Work out the finished part from the listing and answer in its coordinate system (mm). Face numbers are marked on the shaded views. Round coordinates to 2 decimals unless told otherwise and drop trailing zeros. Loops run counter-clockwise (first coordinate to the right, second up) from the corner with the lowest first, then second, coordinate; pieces in that order, holes last.
Autodesk Inventor part; units mm, degrees
ref_plane "YZ Plane" through (0, 0, 0) normal (1, 0, 0) x (0, 1, 0)
ref_plane "XZ Plane" through (0, 0, 0) normal (0, 1, 0) x (-1, 0, 0)
ref_plane "XY Plane" through (0, 0, 0) normal (0, 0, 1) x (1, 0, 0)
sketch "Sketch1" plane through (0, 0, 0) normal (0, 1, 0) x (-1, 0, 0)
  line L0 (-12.5, -5) -> (12.5, -5)
  line L1 (12.5, 0) -> (12.5, 0)
  line L2 (12.5, 5) -> (-12.5, 5)
  line L3 (-12.5, 0) -> (-12.5, 0)
  line L4 (-12.5, -5) -> (12.5, 5) construction
  line L5 (12.5, -5) -> (-12.5, 5) construction
  circle A0 centre (10, 0) radius 1
  circle A1 centre (0, 0) radius 2.5
  line L6 (-12.5, 5) -> (-12.5, -5)
  line L7 (12.5, 5) -> (12.5, -5)
  circle A2 centre (-10, 0) radius 1
  point P0 (0, 0)
  dimension "d0" = 10
  dimension "d1" = 25
  dimension "d3" = 2
  dimension "d4" = 5
  dimension "d6" = 2.5
  dimension "d7" = 5
  dimension "d8" = 5
  dimension "d12" = 0
  dimension "d13" = 2
  dimension "d14" = 2.5
  dimension "d15" = 5
extrude "Extrusion1" add sketch "Sketch1" along normal blind 5
properties part number "link"
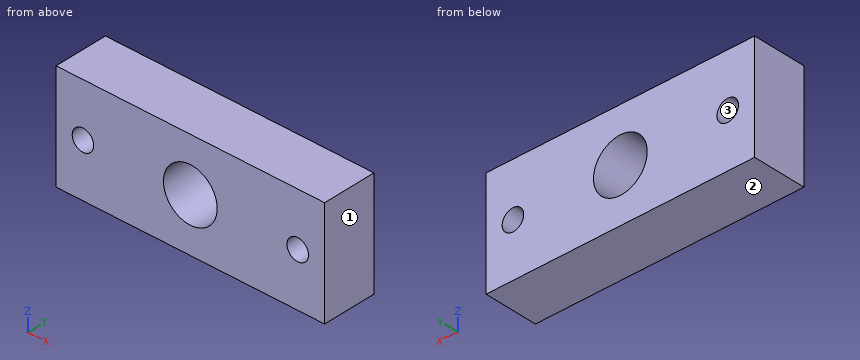
1. Consider probe 1 along Z at (x, y) = (10, 3.55); probe 2 along Z at (x, y) = (0, 1.4); probe 3 along X at (y, z) = (0.4, -2). Determine where each line is inside the solid, lowest interval first.
Answer key:
probe 1: z = -5 to -1, 1 to 5
probe 2: z = -5 to -2.5, 2.5 to 5
probe 3: x = -12.5 to -1.5, 1.5 to 12.5
2. Determine the mould class of the marked faces 1, 2 and 3 for opening direction X: +X half, -X half, draft (parallel to the pull), parting line (faces both ways), or undercut.
Answer key:
face 1: +X half
face 2: draft
face 3: undercut
3. Find section D-D (z = 1.25). Write down the section's boundary in (x, y).
Answer key:
outline: (-12.5, 0) - (-2.17, 0) - (-2.17, 5) - (-12.5, 5) - close; (2.17, 0) - (12.5, 0) - (12.5, 5) - (2.17, 5) - close
4. Find section A-A (x = -1.5). Write down the section's boundary in (y, z), then the cut area to 3 significant figures.
Answer key:
outline: (0, -5) - (5, -5) - (5, -2) - (0, -2) - close; (0, 2) - (5, 2) - (5, 5) - (0, 5) - close
area: 30.0 mm2
5. Find section C-C (y = 0.3). Write down the section's boundary in (x, z), then the cut area to 3 significant figures.
Answer key:
outline: (-12.5, -5) - (12.5, -5) - (12.5, 5) - (-12.5, 5) - close; hole circle Ø2 at (-10, 0); hole circle Ø5 at (0, 0); hole circle Ø2 at (10, 0)
area: 224 mm2
6. Given pin 1 (4.5 mm diameter, centred on x = 0, z = 0, fed in from -Y); pin 2 (5 mm diameter, centred on x = 0.5, z = 2.5, fed in from -Y), each flat-ended and moving along its own axis, determine where each tip first touches the part or whether it passes through.
Answer key:
pin 1: passes through
pin 2: stops at y = 0
7. Find section B-B (z = 0). Write down the section's boundary in (x, y), then the cut area to 3 significant figures.
Answer key:
outline: (-12.5, 0) - (-11, 0) - (-11, 5) - (-12.5, 5) - close; (-9, 0) - (-2.5, 0) - (-2.5, 5) - (-9, 5) - close; (2.5, 0) - (9, 0) - (9, 5) - (2.5, 5) - close; (11, 0) - (12.5, 0) - (12.5, 5) - (11, 5) - close
area: 80.0 mm2
